Geometry: final body of the model. Coordinates: model frame, mm. A direction names the side the tool comes from. Round coordinates to 2 decimals unless told otherwise and drop trailing zeros. Loops run counter-clockwise (first coordinate to the right, second up) from the corner with the lowest first, then second, coordinate; pieces in that order, holes last. Notation, with made-up numbers: (-39.5, 74) -> (18.5, 74) arc R15 cw to (18.5, 96) -> close; hole circle Ø8 at (28.5, 64). An arc over 180 degrees is marked (long way). Answer in a Markdown table with one row per item.
```python
from build123d import *

# Parameters (mm, degrees)
SKETCH1_R           = 9
BOSS_EXTRUDE1_DEPTH = 20
SKETCH2_W           = 20
SKETCH2_H           = 68
BOSS_EXTRUDE5_DEPTH = 60
BOSS_EXTRUDE8_DEPTH = 60
SKETCH23_R          = 34
SKETCH24_R          = 20
SKETCH25_R          = 12
CUT_EXTRUDE12_DEPTH = 148.245543226
CUT_EXTRUDE13_START = 15
CUT_EXTRUDE13_DEPTH = 30
BOSS_EXTRUDE9_DEPTH = 5


with BuildPart() as part:
    # Sketch1 → Boss-Extrude1 (new body)
    with BuildSketch(Plane(origin=(0, 0, 0), x_dir=(1, 0, 0), z_dir=(0, 1, 0))):
        with BuildLine():
            Line((52.5, 45), (-52.5, 45))
            ThreePointArc((-52.5, 45), (-66.642135624, 39.142135624), (-72.5, 25))
            Line((-72.5, 25), (-72.5, -25))
            ThreePointArc((-72.5, -25), (-66.642135624, -39.142135624), (-52.5, -45))
            Line((-52.5, -45), (52.5, -45))
            ThreePointArc((52.5, -45), (66.642135624, -39.142135624), (72.5, -25))
            Line((72.5, -25), (72.5, 25))
            ThreePointArc((72.5, 25), (66.642135624, 39.142135624), (52.5, 45))
        make_face()
        with Locations(Location((-52.5, 25, 0), (0, 0, 270))):
            Circle(SKETCH1_R, mode=Mode.SUBTRACT)
        with Locations(Location((-52.5, -25, 0), (0, 0, 270))):
            Circle(SKETCH1_R, mode=Mode.SUBTRACT)
    extrude(amount=BOSS_EXTRUDE1_DEPTH)

    # Sketch2 → Boss-Extrude5 (add)
    with BuildSketch(Plane(origin=(0, 20, 0), x_dir=(1, 0, 0), z_dir=(0, 1, 0))):
        with Locations((2.5, 0)):
            Rectangle(SKETCH2_W, SKETCH2_H)
    extrude(amount=BOSS_EXTRUDE5_DEPTH)

    # Sketch7 → Boss-Extrude8 (add)
    with BuildSketch(Plane(origin=(0, 20, 0), x_dir=(1, 0, 0), z_dir=(0, 1, 0))):
        with BuildLine():
            Line((12.5, -34), (42.5, -34))
            ThreePointArc((42.5, -34), (71.865680555, 0), (42.5, 34))
            Line((42.5, 34), (12.5, 34))
            Line((12.5, 34), (12.5, -34))
        make_face()
    extrude(amount=BOSS_EXTRUDE8_DEPTH)

    # Sketch23 → Loft1 section 0
    with BuildSketch(Plane(origin=(0, 80, 0), x_dir=(1, 0, 0), z_dir=(0, 1, 0))):
        with Locations((37.5, 0)):
            Circle(SKETCH23_R)
    # Sketch24 → Loft1 section 1
    with BuildSketch(Plane(origin=(0, 120, 0), x_dir=(1, 0, 0), z_dir=(0, 1, 0))):
        with Locations((37.5, 0)):
            Circle(SKETCH24_R)
    loft()

    # Sketch25 → Cut-Extrude12 (cut, through all)
    with BuildSketch(Plane(origin=(0, 120, 0), x_dir=(1, 0, 0), z_dir=(0, 1, 0))):
        with Locations(Location((37.5, 0, 0), (0, 0, 270))):
            Circle(SKETCH25_R)
    extrude(amount=-CUT_EXTRUDE12_DEPTH, mode=Mode.SUBTRACT)

    # Sketch7_2 → Cut-Extrude13 (cut)
    with BuildSketch(Plane(origin=(0, 20, 0), x_dir=(1, 0, 0), z_dir=(0, 1, 0)).offset(CUT_EXTRUDE13_START)):
        with BuildLine():
            Line((12.5, -34), (42.5, -34))
            ThreePointArc((42.5, -34), (71.865680555, 0), (42.5, 34))
            Line((42.5, 34), (12.5, 34))
            Line((12.5, 34), (12.5, -34))
        make_face()
    extrude(amount=CUT_EXTRUDE13_DEPTH, mode=Mode.SUBTRACT)

    # Sketch27 → Boss-Extrude9 (add, symmetric)
    with BuildSketch(Plane.XY):
        Polygon((-7.5, 80), (-7.5, 20), (-72.5, 20), align=None)
    extrude(amount=BOSS_EXTRUDE9_DEPTH, both=True)


solid = part.part
```
Item 1: Cut plane B-B (x = -48). Output: boundary loops of the cut face in (y, z).
Answer:
| item | result |
|---|---|
| outline | (0, -45) -> (20, -45) -> (20, -32.79) -> (0, -32.79) -> close; (0, -17.21) -> (20, -17.21) -> (20, -5) -> (42.62, -5) -> (42.62, 5) -> (20, 5) -> (20, 17.21) -> (0, 17.21) -> close; (0, 32.79) -> (20, 32.79) -> (20, 45) -> (0, 45) -> close |
Item 2: Line query: probe 1 along Z at (x, y) = (-52, 14); probe 2 along Y at (x, z) = (19, 33.5); probe 3 along Y at (x, z) = (34, -18). Output: solid intervals per line, ascending. Write a range as [from, to].
Answer:
| item | result |
|---|---|
| probe 1 | z = [-45, -33.99], [-16.01, 16.01], [33.99, 45] |
| probe 2 | y = [0, 35], [65, 80] |
| probe 3 | y = [0, 35], [65, 120] |
Item 3: Draft query along Z for faces 5 (the face through (-66.486, 9.86, -39.297)), 6 (the face through (-49.797, 9.86, 33.584)), 7 (the face through (72.5, 10, 0)), 8 (the face through (-1, 10, 45)). Return one class per face: pulls with the +Z half, pulls with the -Z half, needs draft (parallel to the pull), parting line crosses it, or undercut.
Answer:
| item | result |
|---|---|
| face 5 | pulls with the -Z half |
| face 6 | undercut |
| face 7 | needs draft |
| face 8 | pulls with the +Z half |
Item 4: Cut plane A-A (y = 11). Output: boundary loops of the cut face in (x, z).
Answer:
| item | result |
|---|---|
| outline | (-72.5, -25) arc R20 ccw to (-52.5, -45) -> (52.5, -45) arc R20 ccw to (72.5, -25) -> (72.5, 25) arc R20 ccw to (52.5, 45) -> (-52.5, 45) arc R20 ccw to (-72.5, 25) -> close; hole circle Ø18 at (-52.5, -25); hole circle Ø18 at (-52.5, 25); hole circle Ø24 at (37.5, 0) |
Item 5: Cut plane D-D (y = 52). Output: boundary loops of the cut face in (x, z).
Answer:
| item | result |
|---|---|
| outline | (-37.83, -5) -> (-7.5, -5) -> (-7.5, -34) -> (12.5, -34) -> (12.5, 34) -> (-7.5, 34) -> (-7.5, 5) -> (-37.83, 5) -> close |
Item 6: Pin query (flat end, axial travel): pin 1 Ø18 at (x, y) = (-30.5, 48) entering from -Z; pin 2 Ø14.5 at (y, z) = (53, 15) entering from -X; pin 3 Ø10 at (y, z) = (99, -22.5) entering from -X; pin 4 Ø6 at (x, z) = (37.5, -6) entering from -Y. Return the tip coordinate at first contact, or that it passes through.
Answer:
| item | result |
|---|---|
| pin 1 | stops at z = -5 |
| pin 2 | stops at x = -7.5 |
| pin 3 | stops at x = 15.9 |
| pin 4 | passes through |
Item 7: Reachability of faces 1 (the face through (71.86, 27.4, 0.69)), 2 (the face through (-7.5, 50, -19)), 3 (the face through (12, 50, 34)), 4 (the face through (-7.5, 50, 20)) from +Z, -Z, +X, -X, +Y, -Y: full face, straight path, thin tool, end or side. Return the list, or none.
Answer:
| item | result |
|---|---|
| face 1 | +X, +Y |
| face 2 | -Z, -X, +Y |
| face 3 | +Z, +X, -X, +Y |
| face 4 | +Z, -X, +Y |
Item 8: Cut plane C-C (z = 0). Count the separate pieces of the cut face and the enclosed holes in it, then the cut area to 3 significant figures.
Answer:
| item | result |
|---|---|
| separate pieces | 3 |
| enclosed holes | 0 |
| area | 7,830 mm² |
